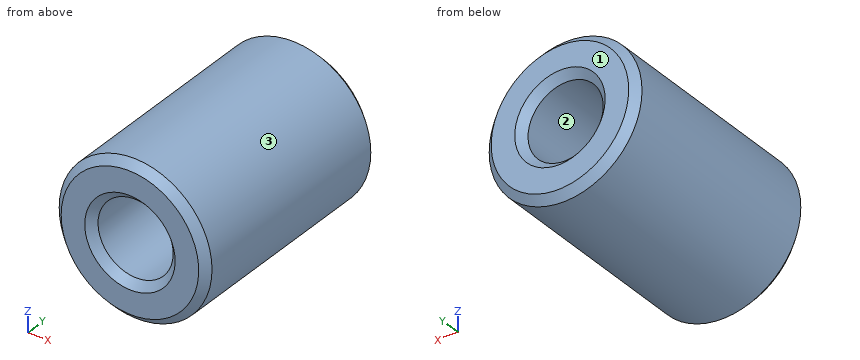
Autodesk Inventor part; units mm, degrees
ref_plane "YZ Plane" through (0, 0, 0) normal (1, 0, 0) x (0, 1, 0)
ref_plane "XZ Plane" through (0, 0, 0) normal (0, 1, 0) x (-1, 0, 0)
ref_plane "XY Plane" through (0, 0, 0) normal (0, 0, 1) x (1, 0, 0)
sketch "Sketch1" plane through (0, 0, 0) normal (0, 1, 0) x (-1, 0, 0)
  circle A0 centre (0, 0) radius 5
  dimension "d0" = 10
extrude "Extrusion1" add sketch "Sketch1" along normal blind 15
hole "Hole1" at (0, 0, 0) direction (0, 1, 0) diameter 4.917 end through all
chamfer "Chamfer1" distance 0.5 angle 45 4 edges at (5, 0, 0) (0, 0, 2.4585) (5, 15, 0) (0, 15, 2.4585)
properties part number "gevindmuffe" material "Steel"
Model file for the job. Use its own axes, mm. Face numbers are marked on the shaded views. Round coordinates to 2 decimals unless told otherwise and drop trailing zeros. Write each loop counter-clockwise with the first axis right and the second up, starting at its lowest first coordinate (ties: lowest second). Pieces come first, ordered by that corner, then holes. Notation, with made-up numbers: M 66,51 L 80,51 A7 cw 80,57 Z; hole C 6,24 d4. An arc over 180 degrees is marked long. Put each result on its own line as item: value.
Item 1: Flat gauge pins, fed straight in: P1, Ø6, axis at y = 3, z = 4, coming from the +X side; P2, Ø4, axis at x = 1, y = 9, coming from the -Z side; P3, Ø2, axis at x = 0.5, z = 1.5, coming from the +Y side; P4, Ø1.5, axis at x = 1.5, y = 3, coming from the +Z side. Where does each tip first touch, or does it go through?
Responses:
P1: x = 4.9
P2: z = -5
P3: y = 14.62
P4: z = 4.94
Item 2: Cut at A-A (x = 0). List the corners of the cut face in (y, z).
Responses:
outline: M 0,-4.5 L 0.5,-5 L 14.5,-5 L 15,-4.5 L 15,-2.96 L 14.5,-2.46 L 0.5,-2.46 L 0,-2.96 Z; M 0,2.96 L 0.5,2.46 L 14.5,2.46 L 15,2.96 L 15,4.5 L 14.5,5 L 0.5,5 L 0,4.5 Z
Item 3: Cut at C-C (y = 7.75). List the corners of the cut face in (x, z), and give its area (3 significant figures).
Responses:
outline: C 0,0 d10; hole C 0,0 d4.92
area: 59.6 mm²
Item 4: Mould opens along Z. For the marked faces 1, 2 and 3 say: +Z half, -Z half, draft (parallel to the pull), parting line (faces both ways), or undercut.
Responses:
face 1: draft
face 2: undercut
face 3: parting line
Item 5: Cut at B-B (z = 0). List the corners of the cut face in (x, y), and give its area (3 significant figures).
Responses:
outline: M -5,0.5 L -4.5,0 L -2.96,0 L -2.46,0.5 L -2.46,14.5 L -2.96,15 L -4.5,15 L -5,14.5 Z; M 2.46,0.5 L 2.96,0 L 4.5,0 L 5,0.5 L 5,14.5 L 4.5,15 L 2.96,15 L 2.46,14.5 Z
area: 75.2 mm²
Item 6: Probe L1, parallel to Z at x = 0, y = 6.75; L2, parallel to Z at x = 0.5, y = 5.5; L3, parallel to X at y = 1, z = -2. List the from-to ranges inside material, lowest first. Write a range as from..to.
Responses:
L1: -5..-2.46, 2.46..5
L2: -4.97..-2.41, 2.41..4.97
L3: -4.58..-1.43, 1.43..4.58
